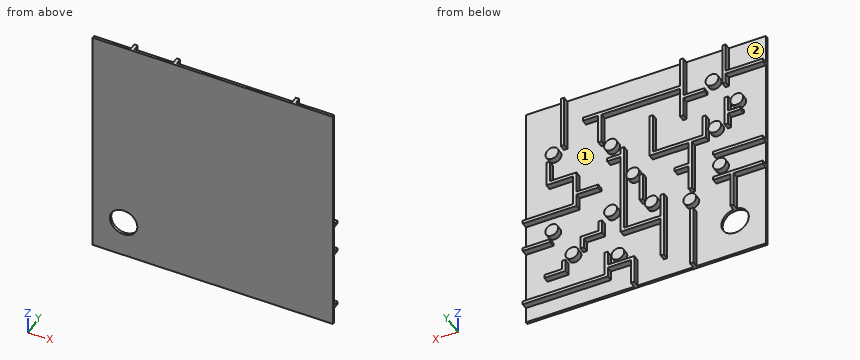
from build123d import *

# Parameters (mm, degrees)
SKETCH1_W           = 280
SKETCH1_H           = 280
SKETCH1_R           = 16
BOSS_EXTRUDE1_DEPTH = 1.5
SKETCH2_R           = 7.5
SKETCH2_W           = 4
SKETCH2_H           = 73.713198053
SKETCH2_W_2         = 58
SKETCH2_H_2         = 4
SKETCH2_H_3         = 64
SKETCH2_W_3         = 32
SKETCH2_H_4         = 34
BOSS_EXTRUDE2_DEPTH = 7


with BuildPart() as part:
    # Sketch1 → Boss-Extrude1 (new, symmetric)
    with BuildSketch(Plane(origin=(0, 0, 0), x_dir=(1, 0, 0), z_dir=(0, 1, 0))):
        Rectangle(SKETCH1_W, SKETCH1_H)
        with Locations(Location((-104, 96, 0), (0, 0, 270))):
            Circle(SKETCH1_R, mode=Mode.SUBTRACT)
    extrude(amount=BOSS_EXTRUDE1_DEPTH, both=True)

    # Sketch2 → Boss-Extrude2 (add)
    with BuildSketch(Plane(origin=(0, 1.5, 0), x_dir=(1, 0, 0), z_dir=(0, 1, 0))):
        with Locations(Location((-54.759044634, 52.982810669, 0), (0, 0, 270))):
            Circle(SKETCH2_R)
        with Locations(Location((-89.473504534, 18.412044198, 0), (0, 0, 270))):
            Circle(SKETCH2_R)
        with Locations(Location((-83.738928303, -33.690548853, 0), (0, 0, 270))):
            Circle(SKETCH2_R)
        with Locations(Location((-109.516269096, -61.269929812, 0), (0, 0, 270))):
            Circle(SKETCH2_R)
        with Locations(Location((-80.69273369, -98.230062392, 0), (0, 0, 270))):
            Circle(SKETCH2_R)
        with Locations(Location((37.587423323, -55.831973409, 0), (0, 0, 270))):
            Circle(SKETCH2_R)
        with Locations(Location((105.9104653, -70.333190482, 0), (0, 0, 270))):
            Circle(SKETCH2_R)
        with Locations(Location((11.819316554, -7.352500668, 0), (0, 0, 270))):
            Circle(SKETCH2_R)
        with Locations(Location((-9.755931913, 39.066973306, 0), (0, 0, 270))):
            Circle(SKETCH2_R)
        with Locations(Location((29.170109307, 94.80128466, 0), (0, 0, 270))):
            Circle(SKETCH2_R)
        with Locations(Location((82.624857116, 73.284632448, 0), (0, 0, 270))):
            Circle(SKETCH2_R)
        with Locations(Location((37.587423323, 33.266850719, 0), (0, 0, 270))):
            Circle(SKETCH2_R)
        with Locations(Location((106.252694304, 33.287862382, 0), (0, 0, 270))):
            Circle(SKETCH2_R)
        with Locations((-57, 103.143400974)):
            Rectangle(SKETCH2_W, SKETCH2_H)
        with BuildLine():
            Line((-140, 37.400802204), (-106, 37.400802204))
            Line((-106, 37.400802204), (-106, 80.125492134))
            ThreePointArc((-106, 80.125492134), (-104, 80), (-102, 80.125492134))
            Line((-102, 80.125492134), (-102, 37.400802204))
            Line((-102, 37.400802204), (-82, 37.400802204))
            Line((-82, 37.400802204), (-82, 33.400802204))
            Line((-82, 33.400802204), (-140, 33.400802204))
            Line((-140, 33.400802204), (-140, 37.400802204))
        make_face()
        Polygon((-140, -100.418377476), (-96.668523278, -100.418377476), (-96.668523278, -88.738640334), (-92.668523278, -88.738640334), (-92.668523278, -140), (-96.668523278, -140), (-96.668523278, -104.418377476), (-140, -104.418377476), align=None)
        with Locations((-111, 1.423286191)):
            Rectangle(SKETCH2_W_2, SKETCH2_H_2)
        Polygon((-47.345115434, -140), (-47.345115434, -90.364557891), (-71.881878867, -90.364557891), (-71.881878867, -86.364557891), (-47.345115434, -86.364557891), (-47.345115434, -63.088559208), (-43.345115434, -63.088559208), (-43.345115434, -100.418377476), (48.027751829, -100.418377476), (48.027751829, -64.371939455), (52.027751829, -64.371939455), (52.027751829, -100.418377476), (69.827851451, -100.418377476), (69.827851451, -104.418377476), (-43.345115434, -104.418377476), (-43.345115434, -140), align=None)
        Polygon((140, 7.737266613), (81.293142587, 7.737266613), (81.293142587, -29.543544834), (112.431248518, -29.543544834), (112.431248518, -59.777272974), (108.431248518, -59.777272974), (108.431248518, -33.543544834), (77.293142587, -33.543544834), (77.293142587, -7.47679166), (52.027751829, -7.47679166), (52.027751829, -3.47679166), (77.293142587, -3.47679166), (77.293142587, 11.737266613), (140, 11.737266613), align=None)
        with Locations((93.622601552, -108)):
            Rectangle(SKETCH2_W, SKETCH2_H_3)
        Polygon((-99.510735812, -32.111868954), (-95.510735812, -32.111868954), (-95.510735812, -68.594238703), (-99.510735812, -68.594238703), (-99.510735812, -49.675826938), (-114.127069846, -49.675826938), (-114.127069846, -45.675826938), (-99.510735812, -45.675826938), align=None)
        with Locations((124, 46.843999527)):
            Rectangle(SKETCH2_W_3, SKETCH2_H_2)
        Polygon((-73.435195895, -53.042459291), (-69.435195895, -53.042459291), (-69.435195895, -27.528186601), (-11.837088751, -27.528186601), (-11.837088751, -76.919702569), (-7.837088751, -76.919702569), (-7.837088751, -23.528186601), (-53.440050937, -23.528186601), (-53.440050937, 4.043094912), (-36.882667743, 4.043094912), (-36.882667743, 8.043094912), (-53.440050937, 8.043094912), (-53.440050937, 38.63118777), (-57.440050937, 38.63118777), (-57.440050937, -23.528186601), (-73.435195895, -23.528186601), align=None)
        Polygon((114.833141636, 94.80128466), (114.833141636, 90.80128466), (94.203549623, 90.80128466), (94.203549623, 79.625492134), (90.203549623, 79.625492134), (90.203549623, 94.80128466), align=None)
        with Locations((1.57904958, 15.009472223)):
            Rectangle(SKETCH2_W, SKETCH2_H_4)
        Polygon((68.742119222, 71), (68.742119222, 59.19860167), (47.447056499, 59.19860167), (47.447056499, 42.554658178), (51.447056499, 42.554658178), (51.447056499, 55.19860167), (72.742119222, 55.19860167), (72.742119222, 71), align=None)
        Polygon((21.727135977, -46.6315684), (25.727135977, -46.6315684), (25.727135977, -38.844500644), (41.459511743, -38.844500644), (41.459511743, -34.844500644), (25.727135977, -34.844500644), (25.727135977, 66.420221849), (-20.87255933, 66.420221849), (-20.87255933, 116.344219933), (-24.87255933, 116.344219933), (-24.87255933, 34.358038326), (-20.87255933, 34.358038326), (-20.87255933, 62.420221849), (21.727135977, 62.420221849), align=None)
        Polygon((140, 116.845058218), (44.841725693, 116.845058218), (44.841725693, 87.65657302), (40.841725693, 87.65657302), (40.841725693, 105.182034885), (9.848778982, 105.182034885), (9.848778982, 140), (13.848778982, 140), (13.848778982, 109.182034885), (40.841725693, 109.182034885), (40.841725693, 120.845058218), (140, 120.845058218), align=None)
    extrude(amount=BOSS_EXTRUDE2_DEPTH)


solid = part.part
CAD build for the part. Positions are in the model's coordinates, mm. Face numbers are marked on the shaded views. Give positions to 0.01 mm unless a question says otherwise; leave off trailing zeros. Put each result on its own line as item: value.
(1) Saw through at A-A (y = 3.25). Count the separate pieces of the cut face and the enclosed holes in it, then the cut area to 3 significant figures.
Working result:
separate pieces: 28
enclosed holes: 0
area: 9,070 mm^2
(2) Pull direction X, two halves, no side cores. Call the marked faces 1 and 2: released by +X, released by -X, zero draft, split by the parting line, or undercut.
Working result:
face 1: undercut
face 2: zero draft
(3) Wall check: L1, parallel to X at y = 2.25, z = 25; L2, parallel to X at y = 6, z = 108.5; L3, parallel to Z at x = 123, y = 7.75. Give the ranges that are in metal, low to high.
Working result:
L1: -73.44 to -7.84, 21.73 to 25.73, 77.29 to 81.29
L2: -96.67 to -92.67, -47.35 to -43.35, 91.62 to 95.62
L3: -120.85 to -116.85, -48.84 to -44.84, -11.74 to -7.74
(4) Drop flat-ended pins along their axis: pin 1 Ø4.5 at (x, y) = (70, 4.5) entering from -Z; pin 2 Ø5.5 at (y, z) = (6, -61.5) entering from +X; pin 3 Ø3 at (y, z) = (5, 5) entering from -X. Give the stop position or say it passes through.
Working result:
pin 1: z = -120.85
pin 2: x = 72.74
pin 3: x = -57.44
